The model under review builds one solid part; all positions refer to its coordinate system, in mm. Round coordinates to 2 decimals unless told otherwise and drop trailing zeros. Write each loop counter-clockwise with the first axis right and the second up, starting at its lowest first coordinate (ties: lowest second). Pieces come first, ordered by that corner, then holes. Notation, with made-up numbers: M 73.5,24 L 79.5,24 A13 cw 79.5,40 Z; hole C -31,5 d11. An arc over 180 degrees is marked long. One line per item, written item: value. Start each with the question number.
1) Take a section at B-B, the plane z = 422.5. Write out the cut boundary in (x, y).
2) Wall thickness on probe 1 along Z at (x, y) = (9, 22); probe 2 along Y at (x, z) = (0, 713); probe 3 along Y at (x, z) = (2, 246.5): over which ranges is each line inside the solid? List them lowest first.
3) Take a section at A-A, the plane x = -9. Write out the cut boundary in (y, z).
4) For P1, Ø1.5, axis at x = 20, z = 497.5, coming from the +Y side; P2, Ø8, axis at x = 15.5, y = 19, coming from the -Z side; P3, Ø8, axis at x = -7.5, z = 843, coming from the -Y side; P4, Ø1, axis at y = -5.5, z = 238.5, coming from the +X side, all flat-tipped, find the tip position at first contact; note any pin that passes through.
5) Mouldability with a two-part tool opening along Z and no side actions: class faces 1 (the face through (13, 18, 406.781)), 2 (the face through (-6, -21, 990.6)), 3 (the face through (-20.157, -15.456, 488.366)) as +Z half, -Z half, draft (parallel to the pull), parting line (faces both ways), or undercut.
from build123d import *

# Parameters (mm, degrees)
SKETCH1_R           = 25.4
SKETCH1_R_2         = 21.261108016
BOSS_EXTRUDE1_DEPTH = 990.6
SKETCH2_W           = 28.624747861
SKETCH2_H           = 25.375038237
SKETCH2_W_2         = 30.891350897
CUT_EXTRUDE1_DEPTH  = 134.112
SKETCH4_W           = 21.111143717
SKETCH4_H           = 28.650837901
SKETCH4_H_2         = 27.348431128
CUT_EXTRUDE3_DEPTH  = 26.416
CUT_EXTRUDE4_DEPTH  = 54.864


with BuildPart() as part:
    # Sketch1 → Boss-Extrude1 (new body)
    with BuildSketch(Plane.XY):
        Circle(SKETCH1_R)
        Circle(SKETCH1_R_2, mode=Mode.SUBTRACT)
    extrude(amount=BOSS_EXTRUDE1_DEPTH)

    # Sketch2 → Cut-Extrude1 (cut)
    with BuildSketch(Plane(origin=(0, 0, 0), x_dir=(0, 0, -1), z_dir=(1, 0, 0))):
        with Locations((-871.475907431, -1.917628622)):
            Rectangle(SKETCH2_W, SKETCH2_H)
        with Locations((-117.451174558, -0.32438411)):
            Rectangle(SKETCH2_W_2, SKETCH2_H)
    extrude(amount=CUT_EXTRUDE1_DEPTH, mode=Mode.SUBTRACT)

    # Sketch4 → Cut-Extrude3 (cut)
    with BuildSketch(Plane(origin=(20.34275841, 31.325100943, 990.6), x_dir=(0.8386705679454252, -0.5446390350150252, 0), z_dir=(0.5446390350150253, 0.8386705679454253, 0))):
        with Locations((1.089203724, 391.007961831)):
            Rectangle(SKETCH4_W, SKETCH4_H)
        with Locations((1.089203724, 597.492816454)):
            Rectangle(SKETCH4_W, SKETCH4_H_2)
    extrude(amount=-CUT_EXTRUDE3_DEPTH, mode=Mode.SUBTRACT)

    # Sketch5 → Cut-Extrude4 (cut)
    with BuildSketch(Plane(origin=(54.696152621, 0, 0), x_dir=(0, 0, -1), z_dir=(1, 0, 0))):
        with BuildLine():
            Line((-504.379993857, 12.412385949), (-486.113069106, 12.412385949))
            ThreePointArc((-486.113069106, 12.412385949), (-482.520966658, 10.924488397), (-481.033069106, 7.332385949))
            Line((-481.033069106, 7.332385949), (-481.033069106, -8.595883791))
            ThreePointArc((-481.033069106, -8.595883791), (-482.520966658, -12.187986239), (-486.113069106, -13.675883791))
            Line((-486.113069106, -13.675883791), (-504.379993857, -13.675883791))
            ThreePointArc((-504.379993857, -13.675883791), (-507.972096305, -12.187986239), (-509.459993857, -8.595883791))
            Line((-509.459993857, -8.595883791), (-509.459993857, 7.332385949))
            ThreePointArc((-509.459993857, 7.332385949), (-507.972096305, 10.924488397), (-504.379993857, 12.412385949))
        make_face()
    extrude(amount=-CUT_EXTRUDE4_DEPTH, mode=Mode.SUBTRACT)


solid = part.part
Checked values:
1. outline: C 0,0 d50.8; hole C 0,0 d42.52
2. probe 1: z = 0 to 379.43, 406.78 to 585.27, 613.92 to 990.6
2. probe 2: y = -25.4 to -21.26, 21.26 to 25.4
2. probe 3: y = -25.32 to -21.17, 21.17 to 25.32
3. outline: M -23.75,0 L -19.26,0 L -19.26,990.6 L -23.75,990.6 Z; M 19.26,0 L 23.75,0 L 23.75,990.6 L 19.26,990.6 Z
4. P1: stops at y = 16.57
4. P2: stops at z = 0
4. P3: stops at y = -25.16
4. P4: stops at x = 24.9
5. face 1: undercut
5. face 2: +Z half
5. face 3: draft
